Part model, mm, in its own coordinate system. Face numbers are marked on the shaded views. A direction names the side the tool comes from. Give positions to 0.01 mm unless a question says otherwise; leave off trailing zeros. Order: outer loops, then holes, each group sorted by start corner. A loop starts at its lowest first (then second) coordinate and runs counter-clockwise, first axis right, second up. Notation, with made-up numbers: (-23.5, 22) - (-12.5, 22) arc R32 ccw to (-12.5, 53) - close; hole circle Ø4 at (32.25, 53.25). An arc over 180 degrees is marked (long way). Use one line per item in the form item = value. Start each with the question number.
1. Pull direction Y, two halves, no side cores. Call the marked faces 3, 4, 5 and 6: +Y half, -Y half, draft (parallel to the pull), parting line (faces both ways), or undercut.
2. Tool access for the marked faces 1 and 2: list every direction of +Z, -Z, +X, -X, +Y, -Y with a clear straight run to the whole face (end or side of a thin tool).
3. Pin check, flat tips, straight feed: P1, Ø1.5, axis at x = -3, y = 17, coming from the -Z side; P2, Ø3.5, axis at x = -4.95, z = -44.845, coming from the +Y side; P3, Ø0.8, axis at x = 1, y = 5.5, coming from the +Z side; P4, Ø4, axis at x = -6.5, y = 37.5, coming from the +Z side. Stop position of each tip, or through.
4. Band-saw the part on B-B, the plane y = 19.5. List the corners of the cut face in (x, z).
5. Drill centre lines: line 1 (Y direction, x = -1.5, z = -26.5); line 2 (Y direction, x = -1.75, z = 3); line 3 (Z direction, x = 8.5, y = 16). Where is each one in solid material? Low to high.
6. Band-saw the part on C-C, the plane x = 4.95. State how many separate pieces and enclosed holes the cut face has, plus the area to 3 significant figures.
7. Band-saw the part on A-A, the plane z = -30.5. List the corners of the cut face in (x, y), plus the area to 3 significant figures.
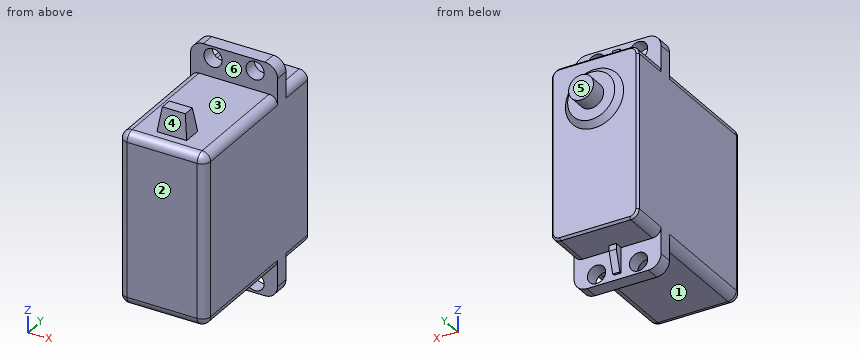
from build123d import *

# Parameters (mm, degrees)
SKETCH1_W           = 40.3
SKETCH1_H           = 40.75
BOSS_EXTRUDE1_DEPTH = 10.25
SKETCH2_R           = 2.93
BOSS_EXTRUDE2_DEPTH = 5.3
SKETCH3_R           = 6.85
BOSS_EXTRUDE3_DEPTH = 1.3
CHAMFER1_SIZE       = 1.3
BOSS_EXTRUDE4_START = 28.36
SKETCH4_W           = 20.5
SKETCH4_H           = 7.2
BOSS_EXTRUDE4_DEPTH = 3.3
CUT_EXTRUDE1_REACH  = 59.997
SKETCH5_R           = 2.15
FILLET1_R           = 2
FILLET2_R           = 3
BOSS_EXTRUDE5_DEPTH = 0.85
CHAMFER2_SIZE       = 0.5
SKETCH8_W           = 7
SKETCH8_H           = 4.33
BOSS_EXTRUDE6_DEPTH = 5.64
BOSS_EXTRUDE6_TAPER = 8


with BuildPart() as part:
    # Sketch1 → Boss-Extrude1 (new, symmetric)
    with BuildSketch(Plane(origin=(0, 0, 0), x_dir=(0, 0, -1), z_dir=(1, 0, 0))):
        with Locations((20.15, 20.375)):
            Rectangle(SKETCH1_W, SKETCH1_H)
    extrude(amount=BOSS_EXTRUDE1_DEPTH, both=True)

    # Sketch2 → Boss-Extrude2 (add)
    with BuildSketch(Plane(origin=(0, 40.75, 0), x_dir=(1, 0, 0), z_dir=(0, 1, 0))):
        with Locations(Location((0, 9.73, 0), (0, 0, 90))):
            Circle(SKETCH2_R)
    extrude(amount=BOSS_EXTRUDE2_DEPTH)

    # Sketch3 → Boss-Extrude3 (add)
    with BuildSketch(Plane(origin=(0, 40.75, 0), x_dir=(1, 0, 0), z_dir=(0, 1, 0))):
        with Locations(Location((0, 9.73, 0), (0, 0, 90))):
            Circle(SKETCH3_R)
    extrude(amount=BOSS_EXTRUDE3_DEPTH)

    # Chamfer1
    chamfer1_edges = [part.edges().sort_by_distance(p)[0] for p in [
        (0, 42.05, -2.88),
    ]]
    chamfer(chamfer1_edges, length=CHAMFER1_SIZE - 0.0001)  # a hair under: the kernel refuses the full size

    # Sketch4 → Boss-Extrude4 (add)
    with BuildSketch(Plane(origin=(0, 0, 0), x_dir=(1, 0, 0), z_dir=(0, 1, 0)).offset(BOSS_EXTRUDE4_START)):
        with Locations((0, -3.6)):
            Rectangle(SKETCH4_W, SKETCH4_H)
        with Locations((0, 43.9)):
            Rectangle(SKETCH4_W, SKETCH4_H)
    extrude(amount=BOSS_EXTRUDE4_DEPTH)

    # Sketch5 → Cut-Extrude1 (cut, up to next)
    with BuildSketch(Plane(origin=(0, 31.66, 0), x_dir=(1, 0, 0), z_dir=(0, 1, 0)), mode=Mode.PRIVATE) as cut_extrude1_sk1:
        with Locations(Location((4.95, -4.545, 0), (0, 0, 270))):
            Circle(SKETCH5_R)
    cut_extrude1_tool1 = extrude(cut_extrude1_sk1.sketch, amount=-CUT_EXTRUDE1_REACH, mode=Mode.PRIVATE) & part.part
    # Sketch5 → Cut-Extrude1 (cut, up to next)
    with BuildSketch(Plane(origin=(0, 31.66, 0), x_dir=(1, 0, 0), z_dir=(0, 1, 0)), mode=Mode.PRIVATE) as cut_extrude1_sk2:
        with Locations(Location((-4.95, -4.545, 0), (0, 0, 270))):
            Circle(SKETCH5_R)
    cut_extrude1_tool2 = extrude(cut_extrude1_sk2.sketch, amount=-CUT_EXTRUDE1_REACH, mode=Mode.PRIVATE) & part.part
    # Sketch5 → Cut-Extrude1 (cut, up to next)
    with BuildSketch(Plane(origin=(0, 31.66, 0), x_dir=(1, 0, 0), z_dir=(0, 1, 0)), mode=Mode.PRIVATE) as cut_extrude1_sk3:
        with Locations(Location((4.95, 44.845, 0), (0, 0, 270))):
            Circle(SKETCH5_R)
    cut_extrude1_tool3 = extrude(cut_extrude1_sk3.sketch, amount=-CUT_EXTRUDE1_REACH, mode=Mode.PRIVATE) & part.part
    # Sketch5 → Cut-Extrude1 (cut, up to next)
    with BuildSketch(Plane(origin=(0, 31.66, 0), x_dir=(1, 0, 0), z_dir=(0, 1, 0)), mode=Mode.PRIVATE) as cut_extrude1_sk4:
        with Locations(Location((-4.95, 44.845, 0), (0, 0, 270))):
            Circle(SKETCH5_R)
    cut_extrude1_tool4 = extrude(cut_extrude1_sk4.sketch, amount=-CUT_EXTRUDE1_REACH, mode=Mode.PRIVATE) & part.part
    add(cut_extrude1_tool1.solids().sort_by_distance((4.95, 31.66, 4.545))[0], mode=Mode.SUBTRACT)
    add(cut_extrude1_tool2.solids().sort_by_distance((-4.95, 31.66, 4.545))[0], mode=Mode.SUBTRACT)
    add(cut_extrude1_tool3.solids().sort_by_distance((4.95, 31.66, -44.845))[0], mode=Mode.SUBTRACT)
    add(cut_extrude1_tool4.solids().sort_by_distance((-4.95, 31.66, -44.845))[0], mode=Mode.SUBTRACT)

    # Fillet1
    fillet1_edges = [part.edges().sort_by_distance(p)[0] for p in [
        (10.25, 14.18, -40.3),
        (-10.25, 14.18, 0),
        (10.25, 14.18, 0),
        (-10.25, 36.205, -40.3),
        (10.25, 36.205, -40.3),
        (10.25, 36.205, 0),
        (-10.25, 14.18, -40.3),
        (-10.25, 0, -20.15),
        (-10.25, 36.205, 0),
        (0, 0, -40.3),
        (0, 0, 0),
        (10.25, 0, -20.15),
    ]]
    fillet(fillet1_edges, radius=FILLET1_R)

    # Fillet2
    fillet2_edges = [part.edges().sort_by_distance(p)[0] for p in [
        (-10.25, 30.01, 7.2),
        (10.25, 30.01, 7.2),
        (10.25, 30.01, -47.5),
        (-10.25, 30.01, -47.5),
    ]]
    fillet(fillet2_edges, radius=FILLET2_R)

    # Sketch7 → Boss-Extrude5 (add, symmetric)
    with BuildSketch(Plane(origin=(0, 0, 0), x_dir=(0, 0, -1), z_dir=(1, 0, 0))):
        Polygon((0, 31.66), (0, 33.57), (-1.3, 33.57), (-5.96, 32.169632375), (-5.96, 31.66), align=None)
    boss_extrude5 = extrude(amount=BOSS_EXTRUDE5_DEPTH, both=True)

    # Mirror1: Boss-Extrude5 across plane
    add(boss_extrude5.mirror(Plane.XY.offset(-20.15)))

    # Chamfer2
    chamfer2_edges = [part.edges().sort_by_distance(p)[0] for p in [
        (10.25, 40.75, -20.15),
        (-10.25, 40.75, -20.15),
        (0, 40.75, 0),
        (0, 40.75, -40.3),
        (9.664213562, 40.75, -39.714213562),
        (-9.664213562, 40.75, -39.714213562),
        (9.664213562, 40.75, -0.585786438),
        (-9.664213562, 40.75, -0.585786438),
    ]]
    chamfer(chamfer2_edges, length=CHAMFER2_SIZE)

    # Sketch8 → Boss-Extrude6 (add)
    with BuildSketch(Plane.XY):
        with Locations((0, 6.005)):
            Rectangle(SKETCH8_W, SKETCH8_H)
    extrude(amount=BOSS_EXTRUDE6_DEPTH, taper=BOSS_EXTRUDE6_TAPER)


solid = part.part
From the geometry:
q1.face_3 = undercut
q1.face_4 = -Y half
q1.face_5 = +Y half
q1.face_6 = undercut
q2.face_1 = -Z, +X, -X, -Y
q2.face_2 = +Z, -Z, +X, -X, -Y
q3.P1 = -40.3
q3.P2 = through
q3.P3 = 5.64
q3.P4 = 0
q4.outline = (-10.25, -38.3) arc R2 ccw to (-8.25, -40.3) - (8.25, -40.3) arc R2 ccw to (10.25, -38.3) - (10.25, -2) arc R2 ccw to (8.25, 0) - (-8.25, 0) arc R2 ccw to (-10.25, -2) - close
q5.line_1 = 0 to 40.75
q5.line_2 = 4.26 to 7.75, 28.36 to 31.66
q5.line_3 = -40.28 to -0.02
q6.separate_pieces = 3
q6.enclosed_holes = 0
q6.area = 1,670 mm²
q7.outline = (-10.25, 2) arc R2 ccw to (-8.25, 0) - (8.25, 0) arc R2 ccw to (10.25, 2) - (10.25, 40.25) - (9.75, 40.75) - (-9.75, 40.75) - (-10.25, 40.25) - close
q7.area = 833 mm²
